For this review, use the dimensioned drawing (mm, ordinates from the lowest corner) and the shaded views. Coordinates: 2 decimals unless noted, no trailing zeros. Write each loop counter-clockwise with the first axis right and the second up, starting at its lowest first coordinate (ties: lowest second). Pieces come first, ordered by that corner, then holes.
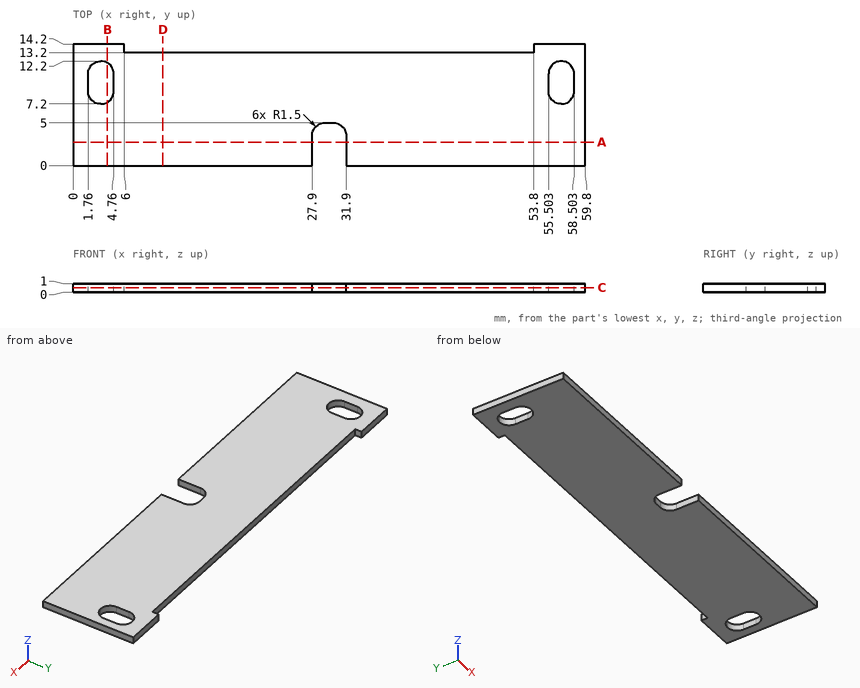
Item 1: To check wall thickness, follow line 1 along X through (y, z) = (10, 0.3); line 2 along Y through (x, z) = (57, 0.8); line 3 along X through (y, z) = (8.25, 0.35). State the ranges of each line that lie inside material, in increasing order.
Solved:
line 1: x = 0 to 1.76, 4.76 to 55.5, 58.5 to 59.8
line 2: y = 0 to 7.2, 12.2 to 14.2
line 3: x = 0 to 1.83, 4.69 to 55.57, 58.43 to 59.8
Item 2: Take a section at D-D, the plane x = 10.5. Write out the cut boundary in (y, z).
Solved:
outline: (0, 0) - (13.2, 0) - (13.2, 1) - (0, 1) - close
Item 3: Take a section at A-A, the plane y = 2.75. Write out the cut boundary in (x, z).
Solved:
outline: (0, 0) - (27.9, 0) - (27.9, 1) - (0, 1) - close; (31.9, 0) - (59.8, 0) - (59.8, 1) - (31.9, 1) - close
Item 4: Take a section at B-B, the plane x = 4. Write out the cut boundary in (y, z) (1 decimal).
Solved:
outline: (0, 0) - (7.4, 0) - (7.4, 1) - (0, 1) - close; (12, 0) - (14.2, 0) - (14.2, 1) - (12, 1) - close
Item 5: Take a section at C-C, the plane z = 0.55. Count the separate pieces of the cut face and the enclosed holes in it, plus the area to 3 significant figures.
Solved:
separate pieces: 1
enclosed holes: 2
area: 756 mm2
